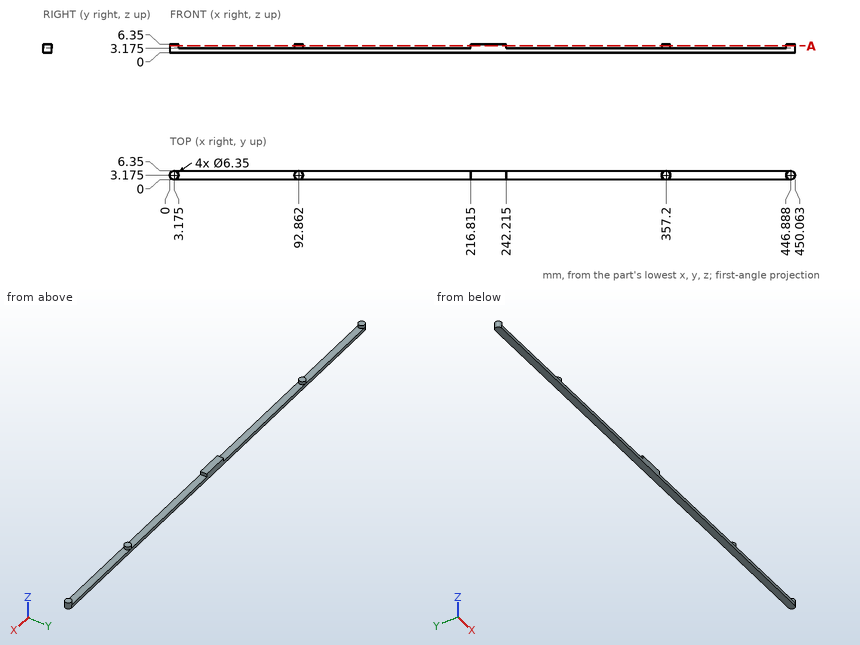
Verification items for this drawing (mm, ordinates from the low corner). Coordinates: 2 decimals unless noted, no trailing zeros. One line per item, written item: value. Start each with the question number.
(1) Material ranges on line 1 (X direction, y = 2.5, z = 4) (1 decimal); line 2 (X direction, y = 1.5, z = 4.25) (1 decimal); line 3 (Z direction, x = 65, y = 2.5) (1 decimal), recorded low to high. Write a range as [from, to].
(2) Depth check by flat-ended pin: P1, Ø1.6, axis at y = 1.5, z = 4.5, coming from the -X side; P2, Ø3, axis at x = 408.5, y = 3.5, coming from the +Z side (3 decimals); P3, Ø1, axis at y = 2, z = 4.5, coming from the +X side. Enter the tip coordinate at first touch or a pass-through.
(3) Cross-section at A-A on z = 5. Count the separate pieces of the cut face and the enclosed holes in it, plus the area to 3 significant figures.
Results below:
1. line 1: x = [0.1, 6.3], [89.8, 96], [216.8, 242.2], [354.1, 360.3], [443.8, 450]
1. line 2: x = [0.5, 5.9], [90.2, 95.6], [216.8, 242.2], [354.5, 359.9], [444.2, 449.6]
1. line 3: z = [0, 3.2]
2. P1: stops at x = 0.12
2. P2: stops at z = 3.175
2. P3: stops at x = 449.99
3. separate pieces: 5
3. enclosed holes: 0
3. area: 288 mm2
